Verification items for the finished model (mm, model axes). Face numbers are marked on the shaded views. A direction names the side the tool comes from. Coordinates: 2 decimals unless noted, no trailing zeros.
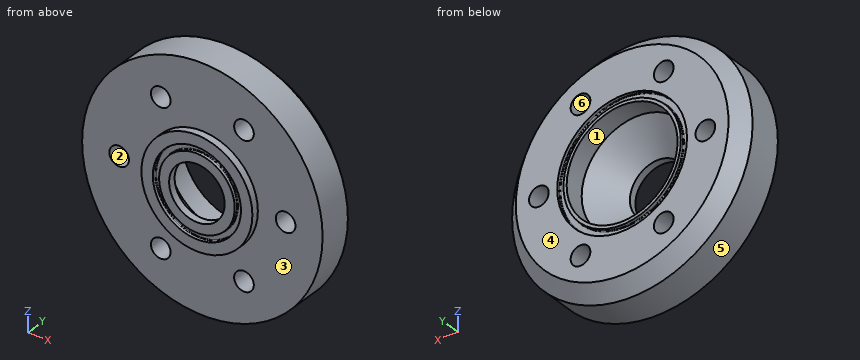
Autodesk Inventor part; units mm, degrees
ref_plane "YZ Plane" through (0, 0, 0) normal (1, 0, 0) x (0, 1, 0)
ref_plane "XZ Plane" through (0, 0, 0) normal (0, 1, 0) x (-1, 0, 0)
ref_plane "XY Plane" through (0, 0, 0) normal (0, 0, 1) x (1, 0, 0)
sketch "Sketch1" plane through (0, 0, 0) normal (0, 0, 1) x (1, 0, 0)
  line L0 (9.525, 0) -> (19.05, 0)
  line L1 (41.275, 19.05) -> (19.05, 19.05)
  line L2 (19.05, 19.05) -> (19.05, 12.065)
  line L3 (19.05, 12.065) -> (9.525, 2.54)
  line L4 (9.525, 2.54) -> (9.525, 0)
  line L5 (0, -3.81) -> (0, 22.86)
  line L6 (19.05, 0) -> (19.05, 2.54)
  line L7 (19.05, 2.54) -> (41.275, 2.54)
  line L8 (41.275, 2.54) -> (41.275, 19.05)
  point P0 (0, 0)
  dimension "d37" = 45
  dimension "d40" = 2.54
  dimension "d57" = 19.05
  dimension "d58" = 9.525
  dimension "d59" = 19.05
  dimension "d60" = 41.275
  dimension "d61" = 2.54
  dimension "d62" = 19.05
revolve "Revolution1" add sketch "Sketch1" angle 360 about axis through (0, -10, 0) along (0, 1, 0)
sketch "Sketch4" plane through (0, 0, 0) normal (0, -1, 0) x (1, 0, 0)
  point P0 (0, 0)
  point P1 (-28.575, 0)
  dimension "d50" = 28.575
hole "Hole2" at (-28.575, 0, 0) direction (0, 1, 0) diameter 6.7564 end through all
pattern_circular "Circular Pattern3" count 6 over 360 about axis through (0, 1.27, 0) along (0, -1, 0) of "Hole2"
chamfer "Chamfer3" distance 4.7625 angle 45 1 edges at (-41.275, 19.05, 0)
sketch "Sketch8" plane through (0, 0, 0) normal (0, 0, 1) x (1, 0, 0)
  line L0 (-22.2758, 19.05) -> (-20.1422, 19.05)
  line L1 (-20.1422, 19.05) -> (-20.1422, 18.034)
  line L2 (-20.3962, 17.78) -> (-22.0218, 17.78)
  line L3 (-22.2758, 18.034) -> (-22.2758, 19.05)
  line L4 (0, -5.1288) -> (0, 30.7731)
  arc A0 (-22.2758, 18.034) -> (-22.0218, 17.78) centre (-22.0218, 18.034) ccw
  arc A1 (-20.3962, 17.78) -> (-20.1422, 18.034) centre (-20.3962, 18.034) ccw
  line L5 (-19.05, 19.05) -> (19.05, 19.05)
  point P0 (0, 0)
  point P1 (-22.2758, 17.78)
  dimension "d88" = 1.27
  dimension "d90" = 22.2758
  dimension "d91" = 2.1336
  dimension "d92" = 0.254
  dimension "d93" = 0.254
  dimension "d94" = 0
revolve "Revolution5" cut sketch "Sketch8" angle 360 about axis through (0, -10, 0) along (0, 1, 0)
sketch "Sketch9" plane through (0, 0, 0) normal (0, 0, 1) x (1, 0, 0)
  line L0 (-14.8717, 1.27) -> (-13.2461, 1.27)
  line L1 (-12.9921, 1.016) -> (-12.9921, 0)
  line L2 (-12.9921, 0) -> (-15.1257, 0)
  line L3 (-15.1257, 0) -> (-15.1257, 1.016)
  arc A0 (-14.8717, 1.27) -> (-15.1257, 1.016) centre (-14.8717, 1.016) ccw
  arc A1 (-12.9921, 1.016) -> (-13.2461, 1.27) centre (-13.2461, 1.016) ccw
  line L4 (0, -3.81) -> (0, 22.86)
  line L5 (0, -15.7794) -> (0, 28.2703) construction
  point P0 (0, 0)
  dimension "d96" = 15.1257
  dimension "d97" = 0.254
  dimension "d98" = 1.27
  dimension "d99" = 2.1336
revolve "Revolution6" cut sketch "Sketch9" angle 360 about axis through (0, -10, 0) along (0, 1, 0)
properties part number "ODSY-0003-202" material "Aluminum 6061"
1. Draft check along Z on the marked faces 4, 5 and 6. Enter one of: pulls with the +Z half, pulls with the -Z half, needs draft (parallel to the pull), parting line crosses it, or undercut.
2. Tool access check on the marked faces 1, 2 and 3. Record the directions out of +Z, -Z, +X, -X, +Y, -Y that give a thin tool (end or side, any length) a straight path to the whole face; none if there is none.
3. Sectioned sample at A-A, the plane y = 7.75. Give the number of separate pieces and of enclosed holes in the cut face, and give its area (3 significant figures).
4. Material ranges on L1, parallel to Z at x = 0, y = 0.65 (3 decimals); L2, parallel to X at y = 1.55, z = 0 (3 decimals); L3, parallel to Z at x = 0, y = 18.6, recorded low to high.
5. Gauge pin test, flat ends, axial feed: P1, Ø11.5, axis at x = 0, z = 0, coming from the +Y side; P2, Ø8, axis at x = 14.29, z = -24.75, coming from the -Y side; P3, Ø10, axis at x = 12, z = 5, coming from the +Y side (3 decimals); P4, Ø6, axis at y = 3, z = 32, coming from the +X side. Record the tip position at first contact, or that the pin passes through.
Outcome:
1. face 4: needs draft
1. face 5: parting line crosses it
1. face 6: undercut
2. face 1: +Y
2. face 2: +Y, -Y
2. face 3: -Y
3. separate pieces: 1
3. enclosed holes: 7
3. area: 4,450 mm2
4. L1: z = -19.05 to -15.126, -12.992 to -9.525, 9.525 to 12.992, 15.126 to 19.05
4. L2: x = -19.05 to -9.525, 9.525 to 19.05
4. L3: z = -36.96 to -22.28, -20.14 to -19.05, 19.05 to 20.14, 22.28 to 36.96
5. P1: passes through
5. P2: stops at y = 2.54
5. P3: stops at y = 11.015
5. P4: stops at x = 29.37
